Could you check a few things on this drawing? It's one solid part, dimensions in mm from its lowest x, y, z. A direction names the side the tool comes from. Give positions to 0.01 mm unless a question says otherwise; leave off trailing zeros. Order: outer loops, then holes, each group sorted by start corner. A loop starts at its lowest first (then second) coordinate and runs counter-clockwise, first axis right, second up. Notation, with made-up numbers: (81, 62.5) -> (127, 62.5) arc R25 cw to (127, 79.5) -> close; hole circle Ø10 at (-28, 52). An arc over 180 degrees is marked (long way). Answer as a JSON object with one key per item and string values.
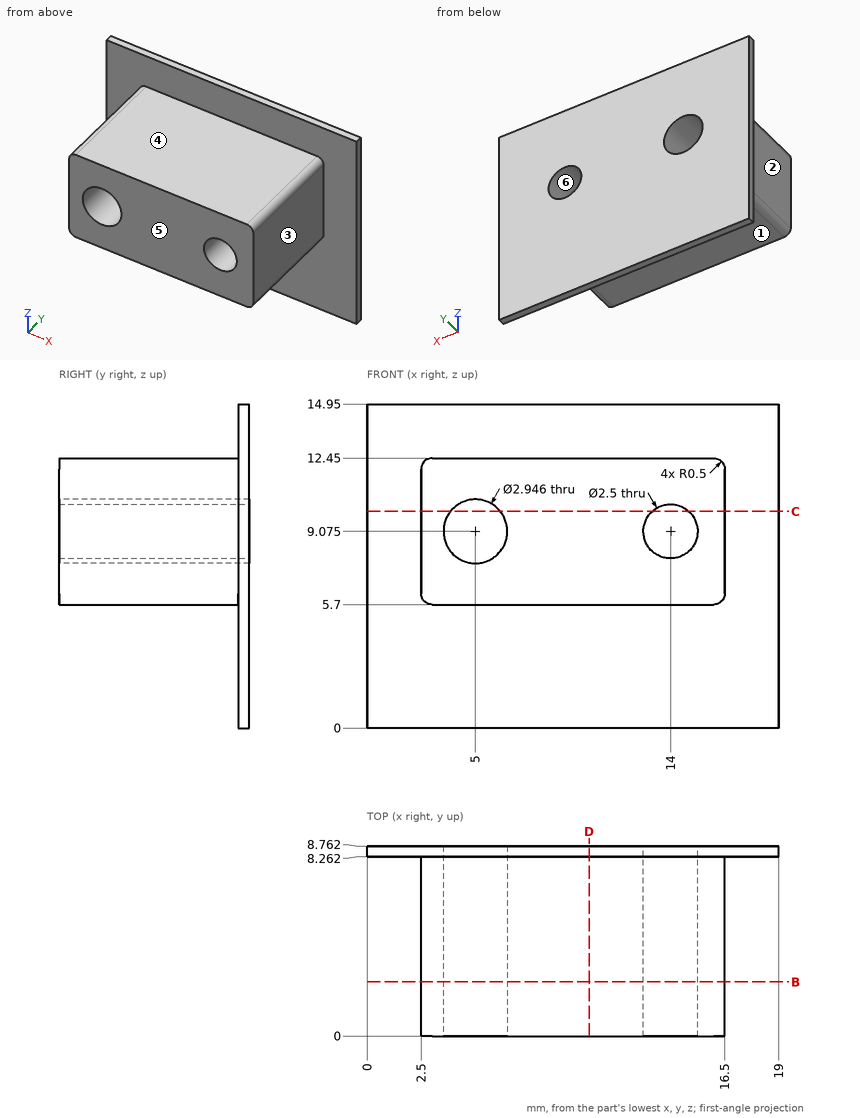
1. Will these pins go through, and if not, where does the flat tip stop? pin 1 Ø2.5 at (x, y) = (7, 5.5) entering from +Z; pin 2 Ø4.5 at (y, z) = (3.5, 7.5) entering from -X; pin 3 Ø2.5 at (x, y) = (10, 2.5) entering from -Z.
Worked answers:
{"pin 1": "z = 12.45", "pin 2": "x = 2.5", "pin 3": "z = 5.7"}
2. Please list where these lines run through material, in increasing order: L1, parallel to Z at x = 5, y = 3; L2, parallel to X at y = 6, z = 9.75; L3, parallel to Y at x = 9.75, z = 13.
Worked answers:
{"L1": "5.7 to 7.6, 10.55 to 12.45", "L2": "2.5 to 3.69, 6.31 to 12.95, 15.05 to 16.5", "L3": "8.26 to 8.76"}
3. For the marked faces 1, 2 and 3, which set-ups out of +Z, -Z, +X, -X, +Y, -Y let a thin tool reach every point of the face, with its end or its side?
Worked answers:
{"face 1": "-Z, +X, -X, -Y", "face 2": "+Z, -Z, -X, -Y", "face 3": "+Z, -Z, +X, -Y"}
4. If we section it at C-C on z = 10: Please give me the cut outline in (x, y).
Worked answers:
{"outline": "(0, 8.26) -> (2.5, 8.26) -> (2.5, 0) -> (3.85, 0) -> (3.85, 8.76) -> (0, 8.76) -> close; (6.15, 0) -> (13.16, 0) -> (13.16, 8.76) -> (6.15, 8.76) -> close; (14.84, 0) -> (16.5, 0) -> (16.5, 8.26) -> (19, 8.26) -> (19, 8.76) -> (14.84, 8.76) -> close"}
5. If we section it at D-D on x = 10.25: Please give me the cut outline in (y, z).
Worked answers:
{"outline": "(0, 5.7) -> (8.26, 5.7) -> (8.26, 0) -> (8.76, 0) -> (8.76, 14.95) -> (8.26, 14.95) -> (8.26, 12.45) -> (0, 12.45) -> close"}
6. If we mould it in two halves opening along Z, with no side actions, what happens to the marked faces 4, 5 and 6? For each: +Z half, -Z half, draft (parallel to the pull), parting line (faces both ways), or undercut.
Worked answers:
{"face 4": "+Z half", "face 5": "draft", "face 6": "undercut"}
7. If we section it at B-B on y = 2.5: Count the separate pieces of the cut face and the enclosed holes in it.
Worked answers:
{"separate pieces": "1", "enclosed holes": "2"}
